Check sheet for the modelled part. Datum: model origin and axes. Units: mm. Face numbers are marked on the shaded views. A direction names the side the tool comes from. Coordinates: 2 decimals unless noted, no trailing zeros. Write each loop counter-clockwise with the first axis right and the second up, starting at its lowest first coordinate (ties: lowest second). Pieces come first, ordered by that corner, then holes. Notation, with made-up numbers: (36.5, 37) -> (95.5, 37) arc R8 ccw to (95.5, 43) -> close; hole circle Ø11 at (39.25, -8). An arc over 180 degrees is marked (long way). Put each result on its own line as item: value.
```python
from build123d import *

# Parameters (mm, degrees)
F0_W            = 43.0059846
F0_H            = 43.0059846
F0_R            = 1.5
F0_R_2          = 11.2530001
F1_DEPTH        = 3.29057
F2_SIZE         = 6.0030106
F4_DEPTH        = 3.29057
F4_COPIES_COUNT = 4


# Not quite as in the source:
# - a pattern or mirror of a feature is missing from the dataset's text; its kind, count and spacing are read off the source's solid


with BuildPart() as f1:
    # F0 (on Top) → F1 (new body)
    with BuildSketch(Plane.XY):
        with Locations((21.5029923, 21.5029923)):
            Rectangle(F0_W, F0_H)
        with Locations((6.0029979, 6.0029979)):
            Circle(F0_R, mode=Mode.SUBTRACT)
        with Locations((21.5029923, 21.5029923)):
            Circle(F0_R_2, mode=Mode.SUBTRACT)
        with Locations((37.0029867, 6.0029979)):
            Circle(F0_R, mode=Mode.SUBTRACT)
        with Locations((6.0029979, 37.0029867)):
            Circle(F0_R, mode=Mode.SUBTRACT)
        with Locations((37.0029867, 37.0029867)):
            Circle(F0_R, mode=Mode.SUBTRACT)
    extrude(amount=F1_DEPTH)

    # F2
    f2_edges = [f1.edges().sort_by_distance(p)[0] for p in [
        (0, 0, 1.645285),
        (0, 43.005985, 1.645285),
        (43.005985, 0, 1.645285),
        (43.005985, 43.005985, 1.645285),
    ]]
    chamfer(f2_edges, length=F2_SIZE)

    # F3 (on face) → F4 (cut, through all)
    with BuildSketch(Plane.XY.offset(3.29057)):
        with BuildLine():
            ThreePointArc((7.2356236023, 32.4027649523), (5.1176370603, 32.3235056996), (3.175, 33.171037571))
            Line((3.175, 33.171037571), (3.175, 9.834947029))
            ThreePointArc((3.175, 9.834947029), (5.1176370603, 10.6824789004), (7.2356236023, 10.6032196477))
            Line((7.2356236023, 10.6032196477), (9.7569670059, 13.1245630513))
            ThreePointArc((9.7569670059, 13.1245630513), (7.0749922, 21.5029923), (9.7569670059, 29.8814215487))
            Line((9.7569670059, 29.8814215487), (7.2356236023, 32.4027649523))
        make_face()
    f4 = extrude(amount=-F4_DEPTH, mode=Mode.SUBTRACT)

    # F4_copies: F4 ×4 about axis
    f4_copies_axis = Axis((21.502992, 21.502992, 0), (0, 0, 1))
    for i in range(1, F4_COPIES_COUNT):
        add(f4.rotate(f4_copies_axis, i * 360 / F4_COPIES_COUNT), mode=Mode.SUBTRACT)


solid = f1.part
```
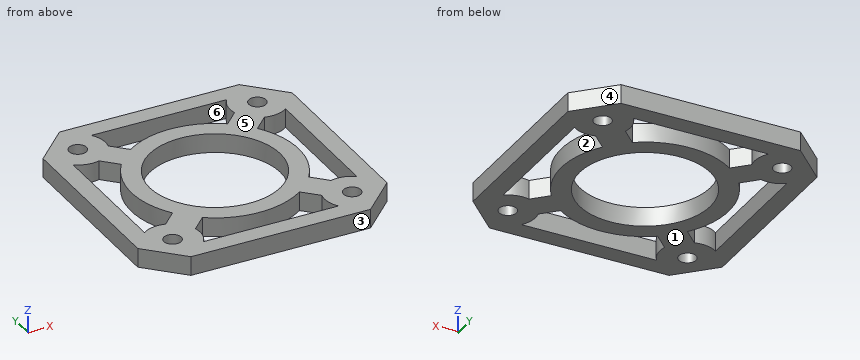
Q1. Mould release check, pull along Y, two halves, no side actions. Record for the marked faces 1, 2, 3 and 4: released by +Y, released by -Y, zero draft, split by the parting line, or undercut.
Recorded:
face 1: zero draft
face 2: undercut
face 3: released by -Y
face 4: released by +Y
Q2. Cross-section at C-C (x = 9). Record the cut outline in (y, z).
Recorded:
outline: (0, 0) -> (12.37, 0) -> (12.37, 3.29) -> (0, 3.29) -> close; (14.3, 0) -> (28.7, 0) -> (28.7, 3.29) -> (14.3, 3.29) -> close; (30.64, 0) -> (43.01, 0) -> (43.01, 3.29) -> (30.64, 3.29) -> close
Q3. Material ranges on line 1 along X through (y, z) = (6, 2); line 2 along X through (y, z) = (22, 1.65) (3 decimals); line 3 along Y through (x, z) = (18, 2.95) (3 decimals), recorded low to high.
Recorded:
line 1: x = 0 to 4.5, 7.5 to 10.77, 32.24 to 35.5, 38.5 to 43
line 2: x = 0 to 3.175, 7.084 to 10.261, 32.745 to 35.922, 39.831 to 43.006
line 3: y = 0 to 3.175, 7.507 to 10.809, 32.197 to 35.499, 39.831 to 43.006
Q4. Depth check by flat-ended pin: P1, Ø2.5, axis at x = 6, y = 6, coming from the -Z side; P2, Ø5, axis at x = 6, y = 37, coming from the -Z side. Enter the tip coordinate at first touch or a pass-through.
Recorded:
P1: passes through
P2: stops at z = 0
Q5. Cross-section at D-D (z = 1.4). State how many separate pieces and enclosed holes the cut face has, plus the area to 3 significant figures.
Recorded:
separate pieces: 1
enclosed holes: 9
area: 923 mm2
Q6. Tool access check on the marked faces 5 and 6. Record the directions out of +Z, -Z, +X, -X, +Y, -Y that give a thin tool (end or side, any length) a straight path to the whole face; none if there is none.
Recorded:
face 5: +Z, +X, -X, +Y, -Y
face 6: +Z, -Z
Q7. Cross-section at A-A (y = 25.5). Record the cut outline in (x, z) (3 decimals).
Recorded:
outline: (0, 0) -> (3.175, 0) -> (3.175, 3.291) -> (0, 3.291) -> close; (7.64, 0) -> (10.984, 0) -> (10.984, 3.291) -> (7.64, 3.291) -> close; (32.022, 0) -> (35.366, 0) -> (35.366, 3.291) -> (32.022, 3.291) -> close; (39.831, 0) -> (43.006, 0) -> (43.006, 3.291) -> (39.831, 3.291) -> close
Q8. Cross-section at B-B (x = 28). Record the cut outline in (y, z) (3 decimals), plus the area to 3 significant figures.
Recorded:
outline: (0, 0) -> (3.175, 0) -> (3.175, 3.291) -> (0, 3.291) -> close; (8.621, 0) -> (12.315, 0) -> (12.315, 3.291) -> (8.621, 3.291) -> close; (30.691, 0) -> (34.385, 0) -> (34.385, 3.291) -> (30.691, 3.291) -> close; (39.831, 0) -> (43.006, 0) -> (43.006, 3.291) -> (39.831, 3.291) -> close
area: 45.2 mm2
